Could you check a few things on this drawing? It's one solid part, dimensions in mm from its lowest x, y, z. Give positions to 0.01 mm unless a question says otherwise; leave off trailing zeros. Order: outer loops, then holes, each group sorted by start corner. A loop starts at its lowest first (then second) coordinate and runs counter-clockwise, first axis right, second up.
(1) Imagine slicing it at A-A, the plane y = 566. Write out the boundary of the cut face in (x, z).
(2) Imagine slicing it at C-C, the plane x = 198. Write out the boundary of the cut face in (y, z), then the cut area to 3 significant figures.
(3) Will this pin go through, and if not, where does the flat tip stop? pin 1 (15 mm diameter, centred on x = 898.5, z = 29.5, fed in from +Y).
(4) Imagine slicing it at B-B, the plane z = 250. Write out the boundary of the cut face in (x, y).
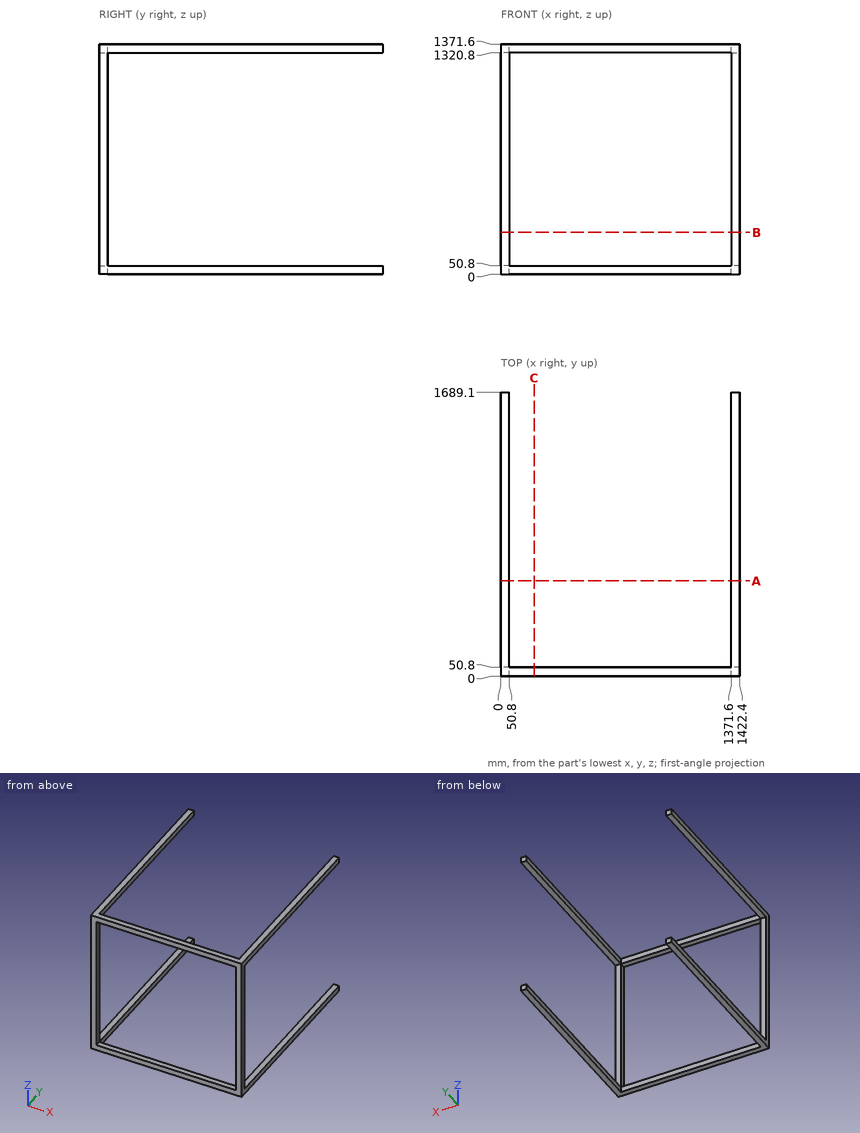
Answer block:
1. outline: (0, 0) - (50.8, 0) - (50.8, 50.8) - (0, 50.8) - close; (0, 1320.8) - (50.8, 1320.8) - (50.8, 1371.6) - (0, 1371.6) - close; (1371.6, 0) - (1422.4, 0) - (1422.4, 50.8) - (1371.6, 50.8) - close; (1371.6, 1320.8) - (1422.4, 1320.8) - (1422.4, 1371.6) - (1371.6, 1371.6) - close
2. outline: (0, 0) - (50.8, 0) - (50.8, 50.8) - (0, 50.8) - close; (0, 1320.8) - (50.8, 1320.8) - (50.8, 1371.6) - (0, 1371.6) - close
2. area: 5,160 mm2
3. pin 1: stops at y = 50.8
4. outline: (0, 0) - (50.8, 0) - (50.8, 50.8) - (0, 50.8) - close; (1371.6, 0) - (1422.4, 0) - (1422.4, 50.8) - (1371.6, 50.8) - close
